from build123d import *


with BuildPart() as part:
    # Sketch2 → Revolve1 (revolve)
    with BuildSketch(Plane.XY):
        with BuildLine():
            Line((-126.767029403, 81.676904789), (-78.228933631, 79.25))
            ThreePointArc((-78.228933631, 79.25), (-60.619483805, 77.84878425), (-43.123035518, 75.413537626))
            ThreePointArc((-43.123035518, 75.413537626), (-41.060447751, 74.831340884), (-39.169286378, 73.823010577))
            ThreePointArc((-39.169286378, 73.823010577), (-35.312933401, 70.206346657), (-32.754159078, 65.579858771))
            Line((-32.754159078, 65.579858771), (-32.056761325, 63.663774193))
            ThreePointArc((-32.056761325, 63.663774193), (-31.860334358, 63.066262055), (-31.701859109, 62.457583237))
            ThreePointArc((-31.701859109, 62.457583237), (-26.081952508, 53.496427146), (-16.098933631, 50))
            Line((-16.098933631, 50), (-16, 50))
            ThreePointArc((-16, 50), (-4.686291501, 54.686291501), (0, 66))
            Line((0, 66), (0, 78.5))
            Line((0, 78.5), (0, 125))
            Line((0, 125), (-132.728933631, 125))
            Line((-132.728933631, 125), (-132.728933631, 97.760533906))
            Line((-132.728933631, 97.760533906), (-132.728933631, 87.760533906))
            ThreePointArc((-132.728933631, 87.760533906), (-132.538632462, 86.803825325), (-131.996700584, 85.992766953))
            Line((-131.996700584, 85.992766953), (-128.409952314, 82.406018683))
            ThreePointArc((-128.409952314, 82.406018683), (-127.656283908, 81.888702675), (-126.767029403, 81.676904789))
        make_face()
    revolve(axis=Axis((0, 125, 0), (-1, 0, 0)))


solid = part.part
Design review of the part built by this model. Coordinates are the model's own, in mm. Coordinates: 2 decimals unless noted, no trailing zeros. Order: outer loops, then holes, each group sorted by start corner. A loop starts at its lowest first (then second) coordinate and runs counter-clockwise, first axis right, second up. Notation, with made-up numbers: (55.25, 49) -> (107.25, 49) arc R18 cw to (107.25, 74) -> close; hole circle Ø11 at (5.5, -18.5). An arc over 180 degrees is marked (long way). Use one line per item in the form item = value. Start each with the question number.
(1) For probe 1 along X at (y, z) = (177, -46.5); probe 2 along Y at (x, z) = (-119, 14.5); probe 3 along Z at (x, y) = (-113, 118), list the stretches that pass through material, from the lowest coordinate up.
(2) Add section C-C on x = -85. State the section outline as (y, z) points.
(3) Add section A-A on z = 0. State the section outline as (x, y) points, plus the area to 3 significant figures.
(4) The part is to be moulded in two halves that separate along Y. For faces 1 (the conical face through (-102.158, 83.844, -17.064)), 2 (the flat face through (0, 126, 1)), say which applies: +Y half, -Y half, draft (parallel to the pull), parting line (faces both ways), or undercut.
(5) Add section B-B on y = 125. State the section outline as (x, z) points, plus the area to 3 significant figures.
(6) Insertion check: pin 1 (6 mm diameter, centred on x = -58.5, z = -33, fed in from +Y); pin 2 (2 mm diameter, centred on x = -113.5, y = 121, fed in from +Z); pin 3 (10 mm diameter, centred on y = 167, z = 11.5, fed in from -X); pin 4 (12 mm diameter, centred on x = -113.5, z = -52, fed in from -Y). Each pin has a flat end and moves straight along its axis. Give the tip position at first contact, or say it passes through.
Answer block:
q1.probe_1 = -27.94 to -4.16
q1.probe_2 = 83.76 to 166.24
q1.probe_3 = -43.45 to 43.45
q2.outline = circle Ø90.82 at (125, 0)
q3.outline = (-132.73, 87.76) arc R2.5 ccw to (-132, 85.99) -> (-128.41, 82.41) arc R2.5 ccw to (-126.77, 81.68) -> (-78.23, 79.25) arc R300 cw to (-43.12, 75.41) arc R10 cw to (-39.17, 73.82) arc R17 cw to (-32.75, 65.58) -> (-32.06, 63.66) arc R10 cw to (-31.7, 62.46) arc R16 ccw to (-16.1, 50) -> (-16, 50) arc R16 ccw to (0, 66) -> (0, 184) arc R16 ccw to (-16, 200) -> (-16.1, 200) arc R16 ccw to (-31.7, 187.54) arc R10 cw to (-32.06, 186.34) -> (-32.75, 184.42) arc R17 cw to (-39.17, 176.18) arc R10 cw to (-43.12, 174.59) arc R300 cw to (-78.23, 170.75) -> (-126.77, 168.32) arc R2.5 ccw to (-128.41, 167.59) -> (-132, 164.01) arc R2.5 ccw to (-132.73, 162.24) -> close
q3.area = 13,900 mm²
q4.face_1 = parting line
q4.face_2 = draft
q5.outline = (-132.73, -37.24) arc R2.5 ccw to (-132, -39.01) -> (-128.41, -42.59) arc R2.5 ccw to (-126.77, -43.32) -> (-78.23, -45.75) arc R300 cw to (-43.12, -49.59) arc R10 cw to (-39.17, -51.18) arc R17 cw to (-32.75, -59.42) -> (-32.06, -61.34) arc R10 cw to (-31.7, -62.54) arc R16 ccw to (-16.1, -75) -> (-16, -75) arc R16 ccw to (0, -59) -> (0, 59) arc R16 ccw to (-16, 75) -> (-16.1, 75) arc R16 ccw to (-31.7, 62.54) arc R10 cw to (-32.06, 61.34) -> (-32.75, 59.42) arc R17 cw to (-39.17, 51.18) arc R10 cw to (-43.12, 49.59) arc R300 cw to (-78.23, 45.75) -> (-126.77, 43.32) arc R2.5 ccw to (-128.41, 42.59) -> (-132, 39.01) arc R2.5 ccw to (-132.73, 37.24) -> close
q5.area = 13,900 mm²
q6.pin_1 = 161.73
q6.pin_2 = 43.9
q6.pin_3 = -132.36
q6.pin_4 = through
